Design review of the part shown in the three views and the two pictorial views. Dimensions are in mm from the part's minimum x, y and z. Give positions to 0.01 mm unless a question says otherwise; leave off trailing zeros. Loops run counter-clockwise (first coordinate to the right, second up) from the corner with the lowest first, then second, coordinate; pieces in that order, holes last. Notation, with made-up numbers: (-20.5, 35.25) - (6.5, 35.25) arc R17 ccw to (6.5, 53.25) - close; hole circle Ø6 at (67, 57). An arc over 180 degrees is marked (long way). Answer as a JSON object with one key per item and string values.
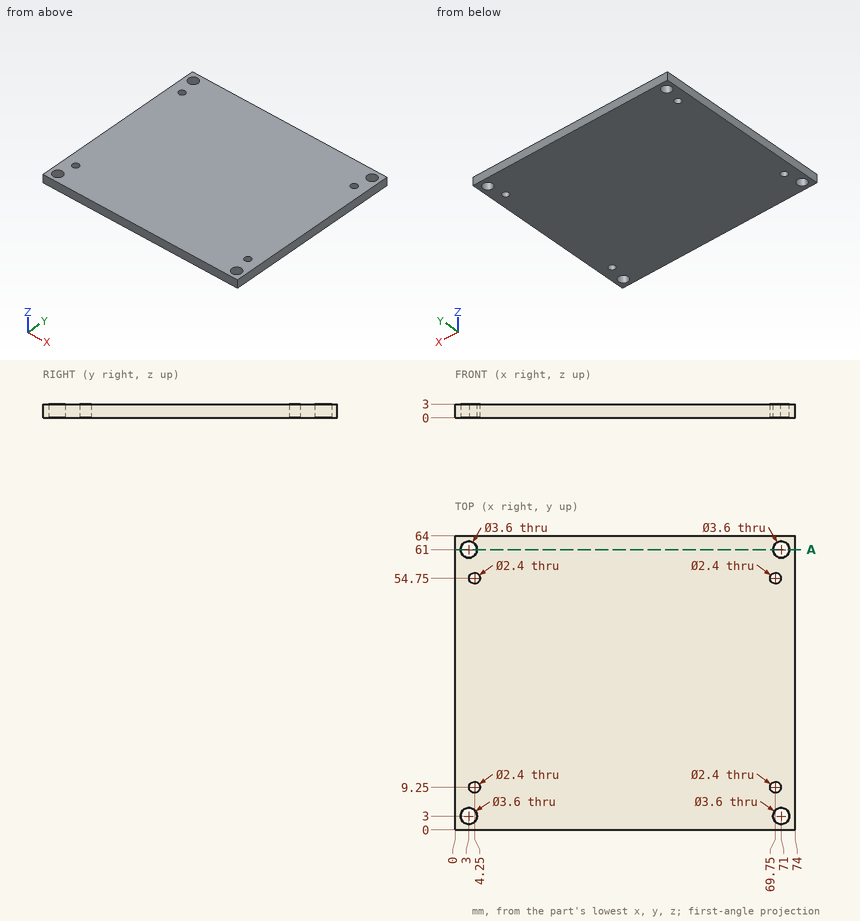
Q1. Consider section A-A, the plane y = 61. State the section outline as (x, z) points, plus the area to 3 significant figures.
Results:
{"outline": "(0, 0) - (1.2, 0) - (1.2, 3) - (0, 3) - close; (4.8, 0) - (69.2, 0) - (69.2, 3) - (4.8, 3) - close; (72.8, 0) - (74, 0) - (74, 3) - (72.8, 3) - close", "area": "200 mm^2"}
Q2. Clearance check with a flat-ended pin moving along its axis: pin 1 Ø2 at (x, y) = (71, 61) entering from +Z. State where the tip first meets the part, or that it passes through.
Results:
{"pin 1": "passes through"}
Q3. To check wall thickness, follow probe 1 along Y at (x, z) = (71, 1.95); probe 2 along X at (y, z) = (61, 2.1); probe 3 along X at (y, z) = (54.75, 1). State the ranges of each line that lie inside material, in increasing order. Write a range as [from, to].
Results:
{"probe 1": "y = [0, 1.2], [4.8, 59.2], [62.8, 64]", "probe 2": "x = [0, 1.2], [4.8, 69.2], [72.8, 74]", "probe 3": "x = [0, 3.05], [5.45, 68.55], [70.95, 74]"}
